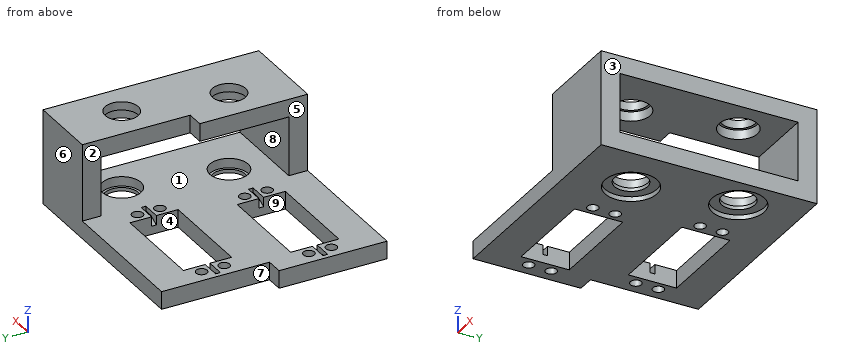
```python
from build123d import *
from OCP.BRepFilletAPI import BRepFilletAPI_MakeChamfer

# Parameters (mm, degrees)
SKETCH1_W           = 37.293223462
SKETCH1_H           = 91.361925627
SKETCH1_R           = 8.1
BOSS_EXTRUDE1_DEPTH = 40
CUT_EXTRUDE1_START  = 8
SKETCH2_W           = 37.293223462
SKETCH2_H           = 25
CUT_EXTRUDE1_DEPTH  = 95.195837814
BOSS_EXTRUDE2_START = -3.5
SKETCH10_R          = 8.1
SKETCH10_R_2        = 7
SKETCH10_R_3        = 10.837031589
BOSS_EXTRUDE2_DEPTH = 3.5
SKETCH11_R          = 8.1
SKETCH11_R_2        = 7
BOSS_EXTRUDE3_DEPTH = 3.5
SKETCH12_W          = 40.9
SKETCH12_H          = 20.4
BOSS_EXTRUDE4_DEPTH = 7.5
CUT_EXTRUDE2_REACH  = 127.125
SKETCH13_R          = 2.3495
SKETCH22_W          = 8
SKETCH22_H          = 2
CUT_EXTRUDE6_DEPTH  = 2
SKETCH14_W          = 37.293223462
SKETCH14_H          = 8
BOSS_EXTRUDE5_DEPTH = 25
CUT_EXTRUDE4_START  = -32.5
SKETCH18_W          = 7.293223462
SKETCH18_H          = 45.680962814
CUT_EXTRUDE4_DEPTH  = 32.5
SKETCH15_R          = 11
CUT_EXTRUDE3_DEPTH  = 2
CHAMFER2_SIZE       = 2
CHAMFER2_SIZE2      = 4.289013841


with BuildPart() as part:
    # Sketch1 → Boss-Extrude1 (new body)
    with BuildSketch(Plane.XY):
        with Locations((3.646611731, 45.680962814)):
            Rectangle(SKETCH1_W, SKETCH1_H)
        with Locations((0, 25)):
            Circle(SKETCH1_R, mode=Mode.SUBTRACT)
        with Locations((7.293223462, 66.361925627)):
            Circle(SKETCH1_R, mode=Mode.SUBTRACT)
    extrude(amount=BOSS_EXTRUDE1_DEPTH)

    # Sketch2 → Cut-Extrude1 (cut, through all)
    with BuildSketch(Plane(origin=(0, 0, 0), x_dir=(1, 0, 0), z_dir=(0, 1, 0)).offset(CUT_EXTRUDE1_START)):
        with Locations((3.646611731, -20)):
            Rectangle(SKETCH2_W, SKETCH2_H)
    extrude(amount=CUT_EXTRUDE1_DEPTH, mode=Mode.SUBTRACT)

    # Sketch10 → Boss-Extrude2 (add)
    # profile 1 of 2: a face of its own
    with BuildSketch(Plane.XY.offset(40).offset(BOSS_EXTRUDE2_START)):
        with Locations(Location((7.293223462, 66.361925627, 0), (0, 0, 180))):
            Circle(SKETCH10_R)
        with Locations((7.293223462, 66.361925627)):
            Circle(SKETCH10_R_2, mode=Mode.SUBTRACT)
    # profile 2 of 2: a face of its own
    with BuildSketch(Plane.XY.offset(40).offset(BOSS_EXTRUDE2_START)):
        with Locations((0, 25)):
            Circle(SKETCH10_R_3)
        with Locations((0, 25)):
            Circle(SKETCH10_R_2, mode=Mode.SUBTRACT)
    extrude(amount=BOSS_EXTRUDE2_DEPTH)

    # Sketch11 → Boss-Extrude3 (add)
    # profile 1 of 2: a face of its own
    with BuildSketch(Plane(origin=(0, 0, 0), x_dir=(-1, 0, 0), z_dir=(0, 0, -1))):
        with Locations((-7.293223462, 66.361925627)):
            Circle(SKETCH11_R)
        with Locations(Location((-7.293223462, 66.361925627, 0), (0, 0, 180))):
            Circle(SKETCH11_R_2, mode=Mode.SUBTRACT)
    # profile 2 of 2: a face of its own
    with BuildSketch(Plane(origin=(0, 0, 0), x_dir=(-1, 0, 0), z_dir=(0, 0, -1))):
        with Locations((0, 25)):
            Circle(SKETCH11_R)
        with Locations(Location((0, 25, 0), (0, 0, 180))):
            Circle(SKETCH11_R_2, mode=Mode.SUBTRACT)
    extrude(amount=-BOSS_EXTRUDE3_DEPTH)

    # Sketch12 → Boss-Extrude4 (add)
    with BuildSketch(Plane(origin=(0, 0, 0), x_dir=(-1, 0, 0), z_dir=(0, 0, -1))):
        Polygon((15, 0), (75.56, 0), (75.56, 45.680962813), (68.266776538, 45.680962813), (68.266776538, 91.361925627), (15, 91.361925627), align=None)
        with Locations((45.11, 25)):
            Rectangle(SKETCH12_W, SKETCH12_H, mode=Mode.SUBTRACT)
        with Locations((37.816776538, 66.361925627)):
            Rectangle(SKETCH12_W, SKETCH12_H, mode=Mode.SUBTRACT)
    extrude(amount=-BOSS_EXTRUDE4_DEPTH)

    # Sketch13 → Cut-Extrude2 (cut, up to next)
    with BuildSketch(Plane(origin=(0, 0, 0), x_dir=(-1, 0, 0), z_dir=(0, 0, -1)), mode=Mode.PRIVATE) as cut_extrude2_sk1:
        with Locations((20.61, 29.75)):
            Circle(SKETCH13_R)
    cut_extrude2_tool1 = extrude(cut_extrude2_sk1.sketch, amount=-CUT_EXTRUDE2_REACH, mode=Mode.PRIVATE) & part.part
    # Sketch13 → Cut-Extrude2 (cut, up to next)
    with BuildSketch(Plane(origin=(0, 0, 0), x_dir=(-1, 0, 0), z_dir=(0, 0, -1)), mode=Mode.PRIVATE) as cut_extrude2_sk2:
        with Locations((20.61, 20.25)):
            Circle(SKETCH13_R)
    cut_extrude2_tool2 = extrude(cut_extrude2_sk2.sketch, amount=-CUT_EXTRUDE2_REACH, mode=Mode.PRIVATE) & part.part
    # Sketch13 → Cut-Extrude2 (cut, up to next)
    with BuildSketch(Plane(origin=(0, 0, 0), x_dir=(-1, 0, 0), z_dir=(0, 0, -1)), mode=Mode.PRIVATE) as cut_extrude2_sk3:
        with Locations((69.61, 29.75)):
            Circle(SKETCH13_R)
    cut_extrude2_tool3 = extrude(cut_extrude2_sk3.sketch, amount=-CUT_EXTRUDE2_REACH, mode=Mode.PRIVATE) & part.part
    # Sketch13 → Cut-Extrude2 (cut, up to next)
    with BuildSketch(Plane(origin=(0, 0, 0), x_dir=(-1, 0, 0), z_dir=(0, 0, -1)), mode=Mode.PRIVATE) as cut_extrude2_sk4:
        with Locations((69.61, 20.25)):
            Circle(SKETCH13_R)
    cut_extrude2_tool4 = extrude(cut_extrude2_sk4.sketch, amount=-CUT_EXTRUDE2_REACH, mode=Mode.PRIVATE) & part.part
    # Sketch13 → Cut-Extrude2 (cut, up to next)
    with BuildSketch(Plane(origin=(0, 0, 0), x_dir=(-1, 0, 0), z_dir=(0, 0, -1)), mode=Mode.PRIVATE) as cut_extrude2_sk5:
        with Locations((13.316776538, 71.111925627)):
            Circle(SKETCH13_R)
    cut_extrude2_tool5 = extrude(cut_extrude2_sk5.sketch, amount=-CUT_EXTRUDE2_REACH, mode=Mode.PRIVATE) & part.part
    # Sketch13 → Cut-Extrude2 (cut, up to next)
    with BuildSketch(Plane(origin=(0, 0, 0), x_dir=(-1, 0, 0), z_dir=(0, 0, -1)), mode=Mode.PRIVATE) as cut_extrude2_sk6:
        with Locations((13.316776538, 61.611925627)):
            Circle(SKETCH13_R)
    cut_extrude2_tool6 = extrude(cut_extrude2_sk6.sketch, amount=-CUT_EXTRUDE2_REACH, mode=Mode.PRIVATE) & part.part
    # Sketch13 → Cut-Extrude2 (cut, up to next)
    with BuildSketch(Plane(origin=(0, 0, 0), x_dir=(-1, 0, 0), z_dir=(0, 0, -1)), mode=Mode.PRIVATE) as cut_extrude2_sk7:
        with Locations((62.316776538, 71.111925627)):
            Circle(SKETCH13_R)
    cut_extrude2_tool7 = extrude(cut_extrude2_sk7.sketch, amount=-CUT_EXTRUDE2_REACH, mode=Mode.PRIVATE) & part.part
    # Sketch13 → Cut-Extrude2 (cut, up to next)
    with BuildSketch(Plane(origin=(0, 0, 0), x_dir=(-1, 0, 0), z_dir=(0, 0, -1)), mode=Mode.PRIVATE) as cut_extrude2_sk8:
        with Locations((62.316776538, 61.611925627)):
            Circle(SKETCH13_R)
    cut_extrude2_tool8 = extrude(cut_extrude2_sk8.sketch, amount=-CUT_EXTRUDE2_REACH, mode=Mode.PRIVATE) & part.part
    add(cut_extrude2_tool1.solids().sort_by_distance((-20.61, 29.75, 0))[0], mode=Mode.SUBTRACT)
    add(cut_extrude2_tool2.solids().sort_by_distance((-20.61, 20.25, 0))[0], mode=Mode.SUBTRACT)
    add(cut_extrude2_tool3.solids().sort_by_distance((-69.61, 29.75, 0))[0], mode=Mode.SUBTRACT)
    add(cut_extrude2_tool4.solids().sort_by_distance((-69.61, 20.25, 0))[0], mode=Mode.SUBTRACT)
    add(cut_extrude2_tool5.solids().sort_by_distance((-13.316777, 71.111926, 0))[0], mode=Mode.SUBTRACT)
    add(cut_extrude2_tool6.solids().sort_by_distance((-13.316777, 61.611926, 0))[0], mode=Mode.SUBTRACT)
    add(cut_extrude2_tool7.solids().sort_by_distance((-62.316777, 71.111926, 0))[0], mode=Mode.SUBTRACT)
    add(cut_extrude2_tool8.solids().sort_by_distance((-62.316777, 61.611926, 0))[0], mode=Mode.SUBTRACT)

    # Sketch22 → Cut-Extrude6 (cut)
    with BuildSketch(Plane.XY.offset(7.5)):
        with Locations((-62.266776538, 66.361925627)):
            Rectangle(SKETCH22_W, SKETCH22_H)
        with Locations((-13.366776538, 66.361925627)):
            Rectangle(SKETCH22_W, SKETCH22_H)
        with Locations((-20.66, 25)):
            Rectangle(SKETCH22_W, SKETCH22_H)
        with Locations((-69.56, 25)):
            Rectangle(SKETCH22_W, SKETCH22_H)
    extrude(amount=-CUT_EXTRUDE6_DEPTH, mode=Mode.SUBTRACT)

    # Sketch14 → Boss-Extrude5 (add)
    with BuildSketch(Plane.XY.offset(7.5)):
        with Locations((3.646611731, 87.361925627)):
            Rectangle(SKETCH14_W, SKETCH14_H)
    extrude(amount=BOSS_EXTRUDE5_DEPTH)

    # Sketch18 → Cut-Extrude4 (cut)
    with BuildSketch(Plane.XY.offset(40).offset(CUT_EXTRUDE4_START)):
        with Locations((-11.353388269, 68.52144422)):
            Rectangle(SKETCH18_W, SKETCH18_H)
    extrude(amount=CUT_EXTRUDE4_DEPTH, mode=Mode.SUBTRACT)

    # Sketch15 → Cut-Extrude3 (cut)
    with BuildSketch(Plane(origin=(0, 0, 0), x_dir=(-1, 0, 0), z_dir=(0, 0, -1))):
        with Locations((0, 25)):
            Circle(SKETCH15_R)
        with Locations((-7.293223462, 66.361925627)):
            Circle(SKETCH15_R)
    extrude(amount=-CUT_EXTRUDE3_DEPTH, mode=Mode.SUBTRACT)

    # Chamfer2: one chamfer whose edges measure the first distance from different faces: ONE call of the kernel's chamfer builder (chamfer() names one face for all edges)
    chamfer2_edges_1 = [part.edges().sort_by_distance(p)[0] for p in [
        (-65.56, 25, 5.5),
    ]]
    chamfer2_side_1 = [part.faces().sort_by_distance(p)[0] for p in [
        (-65.56, 25, 3.676174497),
    ]]
    chamfer2_edges_2 = [part.edges().sort_by_distance(p)[0] for p in [
        (-24.66, 25, 5.5),
    ]]
    chamfer2_side_2 = [part.faces().sort_by_distance(p)[0] for p in [
        (-24.66, 25, 3.676174497),
    ]]
    chamfer2_edges_3 = [part.edges().sort_by_distance(p)[0] for p in [
        (-17.366776538, 66.361925627, 5.5),
    ]]
    chamfer2_side_3 = [part.faces().sort_by_distance(p)[0] for p in [
        (-17.366776538, 66.361925627, 3.676174497),
    ]]
    chamfer2_edges_4 = [part.edges().sort_by_distance(p)[0] for p in [
        (-58.266776538, 66.361925627, 5.5),
    ]]
    chamfer2_side_4 = [part.faces().sort_by_distance(p)[0] for p in [
        (-58.266776538, 66.361925627, 3.676174497),
    ]]
    chamfer2 = BRepFilletAPI_MakeChamfer(part.part.solid().wrapped)
    for e in chamfer2_edges_1:
        chamfer2.Add(CHAMFER2_SIZE, CHAMFER2_SIZE2, e.wrapped, chamfer2_side_1[0].wrapped)  # the first distance lies on this face
    for e in chamfer2_edges_2:
        chamfer2.Add(CHAMFER2_SIZE, CHAMFER2_SIZE2, e.wrapped, chamfer2_side_2[0].wrapped)  # the first distance lies on this face
    for e in chamfer2_edges_3:
        chamfer2.Add(CHAMFER2_SIZE, CHAMFER2_SIZE2, e.wrapped, chamfer2_side_3[0].wrapped)  # the first distance lies on this face
    for e in chamfer2_edges_4:
        chamfer2.Add(CHAMFER2_SIZE, CHAMFER2_SIZE2, e.wrapped, chamfer2_side_4[0].wrapped)  # the first distance lies on this face
    add(Compound.cast(chamfer2.Shape()), mode=Mode.REPLACE)


solid = part.part
```
Model file for the job. Use its own axes, mm. Face numbers are marked on the shaded views. A direction names the side the tool comes from. Round coordinates to 2 decimals unless told otherwise and drop trailing zeros. Write each loop counter-clockwise with the first axis right and the second up, starting at its lowest first coordinate (ties: lowest second). Pieces come first, ordered by that corner, then holes. Notation, with made-up numbers: (87, 27) - (144, 27) arc R20 cw to (144, 46) - close; hole circle Ø3 at (27.5, 21.5). An arc over 180 degrees is marked (long way). Use CSV: the item, a comma, the result in double quotes. Start each with the question number.
Item 1: Band-saw the part on C-C (y = 6). Write the cut outline in (x, z).
Item 2: Band-saw the part on A-A (x = -51). Write the cut outline in (y, z).
Item 3: Tool access for the marked faces 5, 6, 7, 8 and 9: list every direction of +Z, -Z, +X, -X, +Y, -Y with a clear straight run to the whole face (end or side of a thin tool).
Item 4: Pin check, flat tips, straight feed: P1, Ø2, axis at y = 66.5, z = 6.5, coming from the -X side; P2, Ø4, axis at x = -61.5, y = 71, coming from the +Z side; P3, Ø3, axis at x = -71, z = 6, coming from the +Y side. Stop position of each tip, or through.
Item 5: Two-plate mould, pull along X, no slides. Class the marked faces 1, 2, 3 and 4: released by +X, released by -X, zero draft, split by the parting line, or undercut.
Item 6: Band-saw the part on B-B (z = 12). Write the cut outline in (x, y).
Item 7: Band-saw the part on D-D (z = 35). Write the cut outline in (x, y).
Item 8: Drill centre lines: L1, parallel to Y at x = -20.61, z = 5.25; L2, parallel to Z at x = 12, y = 78; L3, parallel to Y at x = -69.61, z = 4.25. Where is each one in solid material? Low to high. Write a range as [from, to].
Checked values:
1,outline,"(-75.56, 0) - (22.29, 0) - (22.29, 40) - (-15, 40) - (-15, 7.5) - (-75.56, 7.5) - close"
2,outline,"(0, 0) - (14.8, 0) - (14.8, 7.5) - (0, 7.5) - close; (35.2, 0) - (56.16, 0) - (56.16, 7.5) - (35.2, 7.5) - close; (76.56, 0) - (91.36, 0) - (91.36, 7.5) - (76.56, 7.5) - close"
3,face 5,"+Z, -X, +Y, -Y"
3,face 6,"+Z, -Z, +X, -X, +Y"
3,face 7,"+Z, -Z, -X, +Y"
3,face 8,"+X, -X"
3,face 9,"+Z, -Z"
4,P1,"stops at x = -68.27"
4,P2,"stops at z = 7.5"
4,P3,"stops at y = 45.68"
5,face 1,"zero draft"
5,face 2,"released by -X"
5,face 3,"released by +X"
5,face 4,"undercut"
6,outline,"(-15, 0) - (22.29, 0) - (22.29, 8) - (-15, 8) - close; (-7.71, 83.36) - (22.29, 83.36) - (22.29, 91.36) - (-7.71, 91.36) - close"
7,outline,"(-15, 0) - (22.29, 0) - (22.29, 91.36) - (-7.71, 91.36) - (-7.71, 45.68) - (-15, 45.68) - close; hole circle Ø16.2 at (0, 25); hole circle Ø16.2 at (7.29, 66.36)"
8,L1,"y = [0, 17.9], [22.6, 27.4], [32.1, 56.16], [76.56, 91.36]"
8,L2,"z = [0, 7.5], [32.5, 40]"
8,L3,"y = [0, 17.9], [22.6, 27.4], [32.1, 45.68]"
